```python
from build123d import *

# Parameters (mm, degrees)
F0_R     = 1.7
F1_DEPTH = 3
F2_R     = 2
F3_R     = 1.7
F4_DEPTH = 6
F5_R     = 2
F6_R     = 1.7
F7_DEPTH = 3
F8_R     = 2.9
F9_DEPTH = 1.5


with BuildPart() as f1:
    # F0 (on Top) → F1 (new body)
    with BuildSketch(Plane.XY):
        Polygon((-2.5, 2.5), (-2.5, 0), (-2.5, -2.5), (47.5, -2.5), (47.5, 0), (47.5, 2.5), align=None)
        Circle(F0_R, mode=Mode.SUBTRACT)
        with Locations((45, 0)):
            Circle(F0_R, mode=Mode.SUBTRACT)
    extrude(amount=F1_DEPTH)

    # F2
    f2_edges = [f1.edges().sort_by_distance(p)[0] for p in [
        (-2.5, 2.5, 1.5),
        (-2.5, -2.5, 1.5),
        (47.5, 2.5, 1.5),
        (47.5, -2.5, 1.5),
    ]]
    fillet(f2_edges, radius=F2_R)

    # F3 (on face) → F4 (join)
    with BuildSketch(Plane(origin=(0, 0, 0), x_dir=(1, 0, 0), z_dir=(0, 0, -1))):
        with BuildLine():
            Line((42.5, -2.5), (45.5, -2.5))
            ThreePointArc((45.5, -2.5), (46.9142135624, -1.9142135624), (47.5, -0.5))
            Line((47.5, -0.5), (47.5, 0.5))
            ThreePointArc((47.5, 0.5), (46.9142135624, 1.9142135624), (45.5, 2.5))
            Line((45.5, 2.5), (42.5, 2.5))
            Line((42.5, 2.5), (42.5, -2.5))
        make_face()
        with Locations((45, 0)):
            Circle(F3_R, mode=Mode.SUBTRACT)
    extrude(amount=F4_DEPTH)

    # F5
    f5_edges = [f1.edges().sort_by_distance(p)[0] for p in [
        (42.5, 2.5, -3),
        (42.5, -2.5, -3),
    ]]
    fillet(f5_edges, radius=F5_R)

    # F6 (on face) → F7 (join, through all)
    with BuildSketch(Plane.XY.offset(3)):
        with BuildLine():
            ThreePointArc((-0.5, 3.5), (-2.6213203436, 2.6213203436), (-3.5, 0.5))
            Line((-3.5, 0.5), (-3.5, -0.5))
            ThreePointArc((-3.5, -0.5), (-2.6213203436, -2.6213203436), (-0.5, -3.5))
            Line((-0.5, -3.5), (3, -3.5))
            Line((3, -3.5), (3, -2.5))
            Line((3, -2.5), (3, 2.5))
            Line((3, 2.5), (3, 3.5))
            Line((3, 3.5), (-0.5, 3.5))
        make_face()
        Circle(F6_R, mode=Mode.SUBTRACT)
    extrude(amount=-F7_DEPTH)

    # F8 (on face) → F9 (cut)
    with BuildSketch(Plane(origin=(0, 0, 0), x_dir=(1, 0, 0), z_dir=(0, 0, -1))):
        Circle(F8_R)
    extrude(amount=-F9_DEPTH, mode=Mode.SUBTRACT)


solid = f1.part
```
The listing builds one solid part. Answer for the finished solid, in the listing's coordinates (mm). A direction names the side the tool comes from. Give positions to 0.01 mm unless a question says otherwise; leave off trailing zeros. Order: outer loops, then holes, each group sorted by start corner. A loop starts at its lowest first (then second) coordinate and runs counter-clockwise, first axis right, second up. Notation, with made-up numbers: (47, 25.5) - (87, 25.5) arc R23 ccw to (87, 62.5) - close; hole circle Ø5 at (29, -11.5). An arc over 180 degrees is marked (long way). Use one line per item in the form item = value. Start each with the question number.
(1) For faces 5 (the flat face through (3, -3, 2)), 6 (the flat face through (42.5, 0, -3)), 7 (the flat face through (26, 2.5, 1)), determine the directions among +Z, -Z, +X, -X, +Y, -Y from which every point of the face is accessible in a straight line to the end or side of a thin tool.
(2) Consider line 1 (X direction, y = 0, z = 2.5); line 2 (X direction, y = 0, z = 1.1); line 3 (Y direction, x = 0, z = 1.95). Determine where each line is inside the solid, lowest interval first. Write a range as from..to.
(3) Flat-ended cylindrical pins translate along their axes: pin 1 Ø1.5 at (y, z) = (-1.5, -1.5) entering from +X; pin 2 Ø5 at (x, z) = (28.5, -4) entering from -Y; pin 3 Ø1 at (y, z) = (-2.5, 1.5) entering from +X; pin 4 Ø4 at (x, y) = (33, 1) entering from -Z. Find the tip coordinate at first contact, or state that the pin passes through.
(4) A cutting plane is placed at A-A, the plane x = 0. Write down the section's boundary in (y, z), then the cut area to 3 significant figures.
(5) A cutting plane is placed at C-C, the plane y = 0. Write down the section's boundary in (x, z), then the cut area to 3 significant figures.
(6) A cutting plane is placed at D-D, the plane z = -5.5. Write down the section's boundary in (x, y), then the cut area to 3 significant figures.
(7) The mould has two halves that part along Y. Classify faces 1 (the flat face through (26, -2.5, 1)), 2 (the cylindrical face through (43.1, 1.93, -3.04)), 3 (the cylindrical face through (-0.37, -1.66, 2.24)), 4 (the flat face through (47.5, 0, -1)): released by +Y, released by -Y, zero draft, split by the parting line, or undercut.
(8) A cutting plane is placed at B-B, the plane z = 1. Write down the section's boundary in (x, y), then the cut area to 3 significant figures.
Ans:
q1.face_5 = +Z, -Z, +X, -Y
q1.face_6 = -Z, -X, +Y, -Y
q1.face_7 = +Z, -Z, +X, +Y
q2.line_1 = -3.5..-1.7, 1.7..43.3, 46.7..47.5
q2.line_2 = -3.5..-2.9, 2.9..43.3, 46.7..47.5
q2.line_3 = -3.5..-1.7, 1.7..3.5
q3.pin_1 = 47.48
q3.pin_2 = through
q3.pin_3 = 46.82
q3.pin_4 = 0
q4.outline = (-3.5, 0) - (-2.9, 0) - (-2.9, 1.5) - (-1.7, 1.5) - (-1.7, 3) - (-3.5, 3) - close; (1.7, 1.5) - (2.9, 1.5) - (2.9, 0) - (3.5, 0) - (3.5, 3) - (1.7, 3) - close
q4.area = 7.20 mm^2
q5.outline = (-3.5, 0) - (-2.9, 0) - (-2.9, 1.5) - (-1.7, 1.5) - (-1.7, 3) - (-3.5, 3) - close; (1.7, 1.5) - (2.9, 1.5) - (2.9, 0) - (42.5, 0) - (42.5, -6) - (43.3, -6) - (43.3, 3) - (1.7, 3) - close; (46.7, -6) - (47.5, -6) - (47.5, 3) - (46.7, 3) - close
q5.area = 139 mm^2
q6.outline = (42.5, -0.5) arc R2 ccw to (44.5, -2.5) - (45.5, -2.5) arc R2 ccw to (47.5, -0.5) - (47.5, 0.5) arc R2 ccw to (45.5, 2.5) - (44.5, 2.5) arc R2 ccw to (42.5, 0.5) - close; hole circle Ø3.4 at (45, 0)
q6.area = 12.5 mm^2
q7.face_1 = released by -Y
q7.face_2 = released by +Y
q7.face_3 = undercut
q7.face_4 = zero draft
q8.outline = (-3.5, -0.5) arc R3 ccw to (-0.5, -3.5) - (3, -3.5) - (3, -2.5) - (45.5, -2.5) arc R2 ccw to (47.5, -0.5) - (47.5, 0.5) arc R2 ccw to (45.5, 2.5) - (3, 2.5) - (3, 3.5) - (-0.5, 3.5) arc R3 ccw to (-3.5, 0.5) - close; hole circle Ø5.8 at (0, 0); hole circle Ø3.4 at (45, 0)
q8.area = 227 mm^2
